Can you work these out from the model? Positions are in its coordinate system, mm. Face numbers are marked on the shaded views. Give positions to 0.01 mm unless a question says otherwise; leave off trailing zeros. Loops run counter-clockwise (first coordinate to the right, second up) from the corner with the lowest first, then second, coordinate; pieces in that order, holes last. Notation, with made-up numbers: (-3, 14) - (44, 14) arc R24 ccw to (44, 41) - close; hole circle Ø3 at (9.5, 76). An arc over 180 degrees is marked (long way). Answer in a Markdown table with one row per item.
from build123d import *

# Parameters (mm, degrees)
SKETCH1_R           = 12
BOSS_EXTRUDE1_DEPTH = 15
SKETCH2_R           = 5.25
CUT_EXTRUDE1_DEPTH  = 7
SKETCH3_R           = 3.25
CUT_EXTRUDE2_DEPTH  = 24
SKETCH4_W           = 33
SKETCH4_H           = 2.6
CUT_EXTRUDE3_DEPTH  = 31


with BuildPart() as part:
    # Sketch1 → Boss-Extrude1 (new body)
    with BuildSketch(Plane(origin=(0, 0, 0), x_dir=(1, 0, 0), z_dir=(0, 1, 0))):
        with BuildLine():
            ThreePointArc((87.921567416, -1.25), (68, 0), (87.921567416, 1.25))
            Line((87.921567416, 1.25), (100, 1.25))
            Line((100, 1.25), (100, 15))
            Line((100, 15), (-100, 15))
            Line((-100, 15), (-100, -15))
            Line((-100, -15), (100, -15))
            Line((100, -15), (100, -1.25))
            Line((100, -1.25), (87.921567416, -1.25))
        make_face()
        with Locations((-83.5, 0)):
            Circle(SKETCH1_R, mode=Mode.SUBTRACT)
    extrude(amount=BOSS_EXTRUDE1_DEPTH)

    # Sketch2 → Cut-Extrude1 (cut)
    with BuildSketch(Plane(origin=(0, 0, -15), x_dir=(-1, 0, 0), z_dir=(0, 0, -1))):
        with Locations((-93, 7.5)):
            Circle(SKETCH2_R)
    extrude(amount=-CUT_EXTRUDE1_DEPTH, mode=Mode.SUBTRACT)

    # Sketch3 → Cut-Extrude2 (cut, through all)
    with BuildSketch(Plane(origin=(0, 0, -8), x_dir=(-1, 0, 0), z_dir=(0, 0, -1))):
        with Locations((-93, 7.5)):
            Circle(SKETCH3_R)
    extrude(amount=-CUT_EXTRUDE2_DEPTH, mode=Mode.SUBTRACT)

    # Sketch4 → Cut-Extrude3 (cut, through all)
    with BuildSketch(Plane(origin=(0, 0, -15), x_dir=(-1, 0, 0), z_dir=(0, 0, -1))):
        with Locations((83.5, 13.7)):
            Rectangle(SKETCH4_W, SKETCH4_H)
    extrude(amount=-CUT_EXTRUDE3_DEPTH, mode=Mode.SUBTRACT)


solid = part.part
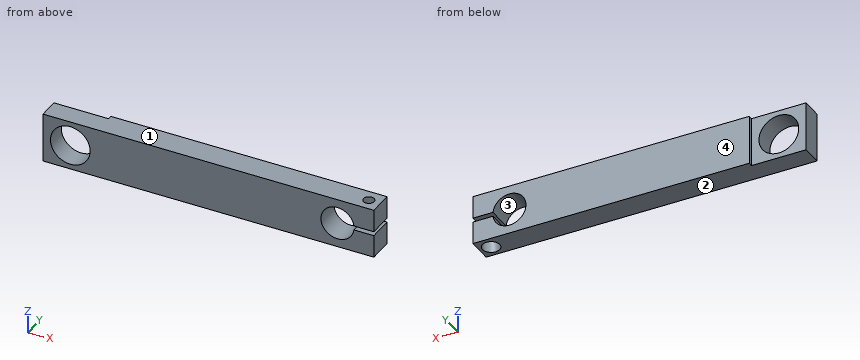
Q1. If we mould it in two halves opening along Z, with no side actions, what happens to the marked faces 1, 2, 3 and 4? For each: released by +Z, released by -Z, zero draft, split by the parting line, or undercut.
Checked values:
| item | result |
|---|---|
| face 1 | released by +Z |
| face 2 | released by -Z |
| face 3 | undercut |
| face 4 | zero draft |
Q2. Imagine slicing it at C-C, the plane x = 84. Write out the boundary of the cut face in (y, z), and give its area (3 significant figures).
Checked values:
| item | result |
|---|---|
| outline | (0, -15) - (15, -15) - (15, -8) - (0, -8) - close; (0, 8) - (15, 8) - (15, 15) - (0, 15) - close |
| area | 210 mm² |
Q3. If I drill on line 1 (X direction, y = 3.5, z = 0); line 2 (X direction, y = 1.5, z = 8); line 3 (Z direction, x = 90.5, y = 2.25), over which ranges is the centre line in solid material (lowest first)? Write a range as [from, to].
Checked values:
| item | result |
|---|---|
| line 1 | x = [-100, -95.5], [-71.5, 68] |
| line 2 | x = [-100, -92.44], [-74.56, 72], [84, 100] |
| line 3 | z = [-15, -1.25], [1.25, 15] |
Q4. For pin 1 (9 mm diameter, centred on x = -77.5, z = 5, fed in from +Y); pin 2 (3.5 mm diameter, centred on x = 94, y = 10, fed in from -Z); pin 3 (0.8 mm diameter, centred on y = 14, z = 7, fed in from -X), each with a flat end and sliding along its axis, tell me the tip position at first contact or that it passes through.
Checked values:
| item | result |
|---|---|
| pin 1 | stops at y = 12.4 |
| pin 2 | stops at z = -8 |
| pin 3 | stops at x = -67 |
Q5. Imagine slicing it at B-B, the plane z = 3. Write out the boundary of the cut face in (x, y).
Checked values:
| item | result |
|---|---|
| outline | (-100, 0) - (-95.12, 0) - (-95.12, 12.4) - (-100, 12.4) - close; (-71.88, 0) - (68.46, 0) - (68.46, 15) - (-67, 15) - (-67, 12.4) - (-71.88, 12.4) - close; (87.54, 0) - (100, 0) - (100, 15) - (87.54, 15) - close; hole circle Ø6.5 at (93, 7.5) |
Q6. Imagine slicing it at D-D, the plane z = -5.25. Write out the boundary of the cut face in (x, y), and give its area (3 significant figures).
Checked values:
| item | result |
|---|---|
| outline | (-100, 0) - (-94.29, 0) - (-94.29, 12.4) - (-100, 12.4) - close; (-72.71, 0) - (69.49, 0) - (69.49, 15) - (-67, 15) - (-67, 12.4) - (-72.71, 12.4) - close; (86.51, 0) - (100, 0) - (100, 15) - (86.51, 15) - close; hole circle Ø6.5 at (93, 7.5) |
| area | 2,360 mm² |
Q7. Imagine slicing it at A-A, the plane y = 7.5. Write out the boundary of the cut face in (x, z).
Checked values:
| item | result |
|---|---|
| outline | (-100, -15) - (87.75, -15) - (87.75, -8) - (89.75, -8) - (89.75, -1.25) - (87.92, -1.25) arc R10 cw (long way) to (87.92, 1.25) - (89.75, 1.25) - (89.75, 15) - (-100, 15) - close; (96.25, -8) - (98.25, -8) - (98.25, -15) - (100, -15) - (100, -1.25) - (96.25, -1.25) - close; (96.25, 1.25) - (100, 1.25) - (100, 15) - (96.25, 15) - close; hole circle Ø24 at (-83.5, 0) |
